The model under review builds one solid part; all positions refer to its coordinate system, in mm. A direction names the side the tool comes from. Give positions to 0.01 mm unless a question says otherwise; leave off trailing zeros. Order: outer loops, then holes, each group sorted by start corner. A loop starts at its lowest first (then second) coordinate and runs counter-clockwise, first axis right, second up. Notation, with made-up numbers: (20.25, 62) - (37.25, 62) arc R23 cw to (37.25, 82) - close; hole circle Ø5 at (-25.5, 80). An arc over 180 degrees is marked (long way). Use a Markdown table: item, result. Add a question column.
```python
from build123d import *

# Parameters (mm, degrees)
F0_W = 20
F0_H = 5


with BuildPart() as f1:
    # F0 (on Top) → F1 (revolve)
    with BuildSketch(Plane.XY):
        Polygon((-10, 0), (-10, 5), (-10, 7.5), (-13, 7.5), (-13, 0), align=None)
        with Locations((0, 2.5)):
            Rectangle(F0_W, F0_H)
        Polygon((10, 7.5), (10, 5), (10, 0), (13, 0), (13, 7.5), align=None)
    revolve(axis=Axis((0, 0, 0), (1, 0, 0)))


solid = f1.part
```
Q1. Wall thickness on probe 1 along X at (y, z) = (-4.5, 4.5); probe 2 along Y at (x, z) = (3.75, -0.25); probe 3 along Y at (x, z) = (-6.25, 4): over which ranges is each line inside the solid? List them lowest first.
Q2. We need section D-D (x = 2.25). Write out the cut boundary in (y, z).
Q3. Draft analysis for pull direction X (two halves, no side actions). For faces 3 (the flat face through (-10, -2, -5)), 4 (the flat face through (-13, 0, 0)), 5 (the cylindrical face through (11.479, -7.493, 0.33)), 6 (the flat face through (13, 0, 0)), state which applies: pulls with the +X half, pulls with the -X half, needs draft (parallel to the pull), parting line crosses it, or undercut.
Q4. Machinability: for faces 1 (the cylindrical face through (-11.521, -7.493, 0.33)), 2 (the flat face through (10, 2, -5)), which of the approach directions +Z, -Z, +X, -X, +Y, -Y give a long, thin tool a straight path to every point of the face, cutting with its end or side? Answer none if there is none.
Q5. Clearance check with flat-ended pins moving along their axes: P1, Ø5, axis at x = 6.5, y = -1.5, coming from the -Z side; P2, Ø3, axis at x = 7, z = -5, coming from the -Y side. State where each tip first meets the part, or that it passes through.
Q6. We need section B-B (y = -5.75). Write out the cut boundary in (x, z).
Q7. We need section A-A (z = 0). Write out the cut boundary in (x, y), plus the area to 3 significant figures.
Here are the results:
| question | item | result |
|---|---|---|
| 1 | probe 1 | -13 to -10, 10 to 13 |
| 1 | probe 2 | -4.99 to 4.99 |
| 1 | probe 3 | -3 to 3 |
| 2 | outline | circle Ø10 at (0, 0) |
| 3 | face 3 | undercut |
| 3 | face 4 | pulls with the -X half |
| 3 | face 5 | needs draft |
| 3 | face 6 | pulls with the +X half |
| 4 | face 1 | +X, -X |
| 4 | face 2 | none |
| 5 | P1 | z = -5 |
| 5 | P2 | y = -3.57 |
| 6 | outline | (-13, -4.82) - (-10, -4.82) - (-10, 4.82) - (-13, 4.82) - close; (10, -4.82) - (13, -4.82) - (13, 4.82) - (10, 4.82) - close |
| 7 | outline | (-13, -7.5) - (-10, -7.5) - (-10, -5) - (10, -5) - (10, -7.5) - (13, -7.5) - (13, 7.5) - (10, 7.5) - (10, 5) - (-10, 5) - (-10, 7.5) - (-13, 7.5) - close |
| 7 | area | 290 mm2 |
